Could you check a few things on this model? Use its own coordinates, in mm. A direction names the side the tool comes from. Coordinates: 2 decimals unless noted, no trailing zeros. Order: outer loops, then holes, each group sorted by start corner. A loop starts at its lowest first (then second) coordinate and runs counter-clockwise, first axis right, second up. Notation, with made-up numbers: (-5, -39) -> (15, -39) arc R7 ccw to (15, -34) -> close; hole circle Ø9 at (72, 81.5). An arc over 180 degrees is marked (long way). Return JSON: item names as keys, results as strings. Group by question number.
from build123d import *

# Parameters (mm, degrees)
SKETCH1_W           = 42
SKETCH1_H           = 50
BOSS_EXTRUDE1_DEPTH = 8
CUT_EXTRUDE1_REACH  = 35.615
SKETCH2_R           = 1.55
SKETCH2_R_2         = 18
SKETCH3_W           = 42
SKETCH3_H           = 50
BOSS_EXTRUDE2_DEPTH = 21
CUT_EXTRUDE2_REACH  = 55.198
SKETCH4_W           = 40
SKETCH4_H           = 19
CUT_EXTRUDE3_REACH  = 45.669
SKETCH6_R           = 2.5


with BuildPart() as part:
    # Sketch1 → Boss-Extrude1 (new body)
    with BuildSketch(Plane(origin=(0, 0, 0), x_dir=(1, 0, 0), z_dir=(0, 1, 0))):
        Rectangle(SKETCH1_W, SKETCH1_H)
    extrude(amount=BOSS_EXTRUDE1_DEPTH)

    # Sketch2 → Cut-Extrude1 (cut, up to next)
    with BuildSketch(Plane(origin=(0, 8, 0), x_dir=(1, 0, 0), z_dir=(0, 1, 0)), mode=Mode.PRIVATE) as cut_extrude1_sk1:
        with Locations(Location((-15.5, 15.5, 0), (0, 0, 270))):
            Circle(SKETCH2_R)
    cut_extrude1_tool1 = extrude(cut_extrude1_sk1.sketch, amount=-CUT_EXTRUDE1_REACH, mode=Mode.PRIVATE) & part.part
    # Sketch2 → Cut-Extrude1 (cut, up to next)
    with BuildSketch(Plane(origin=(0, 8, 0), x_dir=(1, 0, 0), z_dir=(0, 1, 0)), mode=Mode.PRIVATE) as cut_extrude1_sk2:
        with Locations(Location((15.5, 15.5, 0), (0, 0, 270))):
            Circle(SKETCH2_R)
    cut_extrude1_tool2 = extrude(cut_extrude1_sk2.sketch, amount=-CUT_EXTRUDE1_REACH, mode=Mode.PRIVATE) & part.part
    # Sketch2 → Cut-Extrude1 (cut, up to next)
    with BuildSketch(Plane(origin=(0, 8, 0), x_dir=(1, 0, 0), z_dir=(0, 1, 0)), mode=Mode.PRIVATE) as cut_extrude1_sk3:
        with Locations(Location((15.5, -15.5, 0), (0, 0, 270))):
            Circle(SKETCH2_R)
    cut_extrude1_tool3 = extrude(cut_extrude1_sk3.sketch, amount=-CUT_EXTRUDE1_REACH, mode=Mode.PRIVATE) & part.part
    # Sketch2 → Cut-Extrude1 (cut, up to next)
    with BuildSketch(Plane(origin=(0, 8, 0), x_dir=(1, 0, 0), z_dir=(0, 1, 0)), mode=Mode.PRIVATE) as cut_extrude1_sk4:
        with Locations(Location((-15.5, -15.5, 0), (0, 0, 270))):
            Circle(SKETCH2_R)
    cut_extrude1_tool4 = extrude(cut_extrude1_sk4.sketch, amount=-CUT_EXTRUDE1_REACH, mode=Mode.PRIVATE) & part.part
    # Sketch2 → Cut-Extrude1 (cut, up to next)
    with BuildSketch(Plane(origin=(0, 8, 0), x_dir=(1, 0, 0), z_dir=(0, 1, 0)), mode=Mode.PRIVATE) as cut_extrude1_sk5:
        with Locations(Location((0, 0, 0), (0, 0, 270))):
            Circle(SKETCH2_R_2)
    cut_extrude1_tool5 = extrude(cut_extrude1_sk5.sketch, amount=-CUT_EXTRUDE1_REACH, mode=Mode.PRIVATE) & part.part
    add(cut_extrude1_tool1.solids().sort_by_distance((-15.5, 8, -15.5))[0], mode=Mode.SUBTRACT)
    add(cut_extrude1_tool2.solids().sort_by_distance((15.5, 8, -15.5))[0], mode=Mode.SUBTRACT)
    add(cut_extrude1_tool3.solids().sort_by_distance((15.5, 8, 15.5))[0], mode=Mode.SUBTRACT)
    add(cut_extrude1_tool4.solids().sort_by_distance((-15.5, 8, 15.5))[0], mode=Mode.SUBTRACT)
    add(cut_extrude1_tool5.solids().sort_by_distance((0, 8, 0))[0], mode=Mode.SUBTRACT)

    # Sketch3 → Boss-Extrude2 (add)
    with BuildSketch(Plane(origin=(0, 0, 0), x_dir=(1, 0, 0), z_dir=(0, 1, 0))):
        Rectangle(SKETCH3_W, SKETCH3_H)
    extrude(amount=-BOSS_EXTRUDE2_DEPTH)

    # Sketch4 → Cut-Extrude2 (cut, up to next)
    with BuildSketch(Plane.ZY.offset(21), mode=Mode.PRIVATE) as cut_extrude2_sk1:
        with Locations((0, -6.5)):
            Rectangle(SKETCH4_W, SKETCH4_H)
    cut_extrude2_tool1 = extrude(cut_extrude2_sk1.sketch, amount=-CUT_EXTRUDE2_REACH, mode=Mode.PRIVATE) & part.part
    add(cut_extrude2_tool1.solids().sort_by_distance((-21, -6.5, 0))[0], mode=Mode.SUBTRACT)

    # Sketch6 → Cut-Extrude3 (cut, up to next)
    with BuildSketch(Plane(origin=(0, -21, 0), x_dir=(-1, 0, 0), z_dir=(0, -1, 0)), mode=Mode.PRIVATE) as cut_extrude3_sk1:
        with Locations(Location((-15, 15, 0), (0, 0, 90))):
            Circle(SKETCH6_R)
    cut_extrude3_tool1 = extrude(cut_extrude3_sk1.sketch, amount=-CUT_EXTRUDE3_REACH, mode=Mode.PRIVATE) & part.part
    # Sketch6 → Cut-Extrude3 (cut, up to next)
    with BuildSketch(Plane(origin=(0, -21, 0), x_dir=(-1, 0, 0), z_dir=(0, -1, 0)), mode=Mode.PRIVATE) as cut_extrude3_sk2:
        with Locations(Location((15, 15, 0), (0, 0, 90))):
            Circle(SKETCH6_R)
    cut_extrude3_tool2 = extrude(cut_extrude3_sk2.sketch, amount=-CUT_EXTRUDE3_REACH, mode=Mode.PRIVATE) & part.part
    # Sketch6 → Cut-Extrude3 (cut, up to next)
    with BuildSketch(Plane(origin=(0, -21, 0), x_dir=(-1, 0, 0), z_dir=(0, -1, 0)), mode=Mode.PRIVATE) as cut_extrude3_sk3:
        with Locations(Location((15, -15, 0), (0, 0, 90))):
            Circle(SKETCH6_R)
    cut_extrude3_tool3 = extrude(cut_extrude3_sk3.sketch, amount=-CUT_EXTRUDE3_REACH, mode=Mode.PRIVATE) & part.part
    # Sketch6 → Cut-Extrude3 (cut, up to next)
    with BuildSketch(Plane(origin=(0, -21, 0), x_dir=(-1, 0, 0), z_dir=(0, -1, 0)), mode=Mode.PRIVATE) as cut_extrude3_sk4:
        with Locations(Location((-15, -15, 0), (0, 0, 90))):
            Circle(SKETCH6_R)
    cut_extrude3_tool4 = extrude(cut_extrude3_sk4.sketch, amount=-CUT_EXTRUDE3_REACH, mode=Mode.PRIVATE) & part.part
    add(cut_extrude3_tool1.solids().sort_by_distance((15, -21, -15))[0], mode=Mode.SUBTRACT)
    add(cut_extrude3_tool2.solids().sort_by_distance((-15, -21, -15))[0], mode=Mode.SUBTRACT)
    add(cut_extrude3_tool3.solids().sort_by_distance((-15, -21, 15))[0], mode=Mode.SUBTRACT)
    add(cut_extrude3_tool4.solids().sort_by_distance((15, -21, 15))[0], mode=Mode.SUBTRACT)


solid = part.part
Q1. I want a section at A-A on y = -10.5. Please give me the cut outline in (x, z), and give its area (3 significant figures).
Q2. I'm going to push flat-ended pins straight in: pin 1 Ø4 at (x, z) = (-15, -15) entering from -Y; pin 2 Ø3 at (x, z) = (15.5, 15.5) entering from +Y; pin 3 Ø6 at (x, z) = (1.5, 10.5) entering from +Y. Where does each tip first touch, or does it pass through?
Q3. I want a section at D-D on x = 0. Please give me the cut outline in (y, z), and give its area (3 significant figures).
Q4. We'd pull the mould along X, two halves only. Please class faces 1 (the flat face through (-21, 3.4, 0.3)), 2 (the flat face through (21, 3.4, 0.3)), 3 (the flat face through (-14.3, 8, -11.5)), 4 (the cylindrical face through (-14.9, -18.5, -12.5)): pulls with the +X half, pulls with the -X half, needs draft (parallel to the pull), parting line crosses it, or undercut.
Q5. I need wall thicknesses on line 1 along X through (y, z) = (-19.3, 15); line 2 along Z through (x, y) = (-10, -12.5); line 3 along Y through (x, z) = (-15, -10.5). Which ranges of each line are inside material? Lowest first, please. Write a range as from..to.
Q6. I want a section at C-C on z = 2. Please give me the cut outline in (x, y), and give its area (3 significant figures).
Q7. On a 3-axis mill with a long thin cutter (end or side, diameter ignored), from which of +Z, -Z, +X, -X, +Y, -Y can I reach the whole of each face in a straight line? I mean faces 5 (the flat face through (0, -6, -25)), 6 (the cylindrical face through (15.1, -18.5, -12.5)), 7 (the flat face through (4, 3, -18)). Say none if no direction works.
Q8. I want a section at B-B on z = -15. Please give me the cut outline in (x, y), and give its area (3 significant figures).
Response values:
{
 "1": {"outline": "(-21, -25) -> (21, -25) -> (21, -20) -> (-21, -20) -> close; (-21, 20) -> (21, 20) -> (21, 25) -> (-21, 25) -> close", "area": "420 mm²"},
 "2": {"pin 1": "stops at y = 3", "pin 2": "passes through", "pin 3": "stops at y = -16"},
 "3": {"outline": "(-21, -25) -> (8, -25) -> (8, -18) -> (3, -18) -> (3, -20) -> (-16, -20) -> (-16, 20) -> (3, 20) -> (3, 18) -> (8, 18) -> (8, 25) -> (-21, 25) -> close", "area": "510 mm²"},
 "4": {"face 1": "pulls with the -X half", "face 2": "pulls with the +X half", "face 3": "needs draft", "face 4": "undercut"},
 "5": {"line 1": "x = -21..-17.5, -12.5..12.5, 17.5..21", "line 2": "z = -25..-20, 20..25", "line 3": "y = -21..-16, 3..8"},
 "6": {"outline": "(-21, -21) -> (21, -21) -> (21, -16) -> (-21, -16) -> close; (-21, 3) -> (-17.89, 3) -> (-17.89, 8) -> (-21, 8) -> close; (17.89, 3) -> (21, 3) -> (21, 8) -> (17.89, 8) -> close", "area": "241 mm²"},
 "7": {"face 5": "-Z, +X, -X, +Y, -Y", "face 6": "-Y", "face 7": "+X, -X"},
 "8": {"outline": "(-21, -21) -> (-17.5, -21) -> (-17.5, -16) -> (-21, -16) -> close; (-21, 3) -> (-16.97, 3) -> (-16.97, 8) -> (-21, 8) -> close; (-14.03, 3) -> (-9.95, 3) -> (-9.95, 8) -> (-14.03, 8) -> close; (-12.5, -21) -> (12.5, -21) -> (12.5, -16) -> (-12.5, -16) -> close; (9.95, 3) -> (14.03, 3) -> (14.03, 8) -> (9.95, 8) -> close; (16.97, 3) -> (21, 3) -> (21, 8) -> (16.97, 8) -> close; (17.5, -21) -> (21, -21) -> (21, -16) -> (17.5, -16) -> close", "area": "241 mm²"}
}
